Can you work these out from the model? Positions are in its coordinate system, mm. Coordinates: 2 decimals unless noted, no trailing zeros. Loops run counter-clockwise (first coordinate to the right, second up) from the corner with the lowest first, then second, coordinate; pieces in that order, holes last.
Autodesk Inventor part; units mm, degrees
ref_plane "BODYS_XY" through (0, 0, 0) normal (1, 0, 0) x (0, 0, -1)
ref_plane "BODYS_YZ" through (0, 0, 0) normal (0, 0, -1) x (0, 1, 0)
ref_plane "BODYS_ZX" through (0, 0, 0) normal (0, 1, 0) x (1, 0, 0)
sketch "__2" plane through (0, 0, 0) normal (1, 0, 0) x (0, 1, 0)
  arc A0 (0.5, 35.5) -> (0, 35) centre (0.5, 35) ccw
  line L0 (0, 35) -> (0, -35)
  arc A1 (0, -35) -> (0.5, -35.5) centre (0.5, -35) ccw
  line L1 (0.5, -35.5) -> (6.3099, -35.5)
  arc A2 (6.3099, -35.5) -> (8.274, -33.877) centre (6.3099, -33.5) ccw
  arc A3 (8.274, -33.877) -> (8.7, -31.581) centre (-167.9972, 0.0159) ccw
  line L2 (8.7, -31.581) -> (8.7, -29.75)
  line L3 (8.7, -29.75) -> (9.051, -29.547)
  arc A4 (9.051, -29.547) -> (9.051, 29.547) centre (-168.0005, 0) ccw
  line L4 (9.051, 29.547) -> (8.7, 29.75)
  line L5 (8.7, 29.75) -> (8.7, 31.581)
  arc A5 (8.7, 31.581) -> (8.274, 33.877) centre (-167.9972, -0.0159) ccw
  arc A6 (8.274, 33.877) -> (6.3099, 35.5) centre (6.3099, 33.5) ccw
  line L6 (6.3099, 35.5) -> (0.5, 35.5)
extrude "Extrusion1" add sketch "__2" along normal blind 597
sketch "__1" plane through (0, 7.18, 0) normal (0, 1, 0) x (1, 0, 0)
  circle A0 centre (8, 30.29) radius 3.25
extrude "Extrusion2" cut sketch "__1" along normal blind 3.52
pattern_linear "Rectangular Pattern1" count 2 spacing 631 along (1, 0, 0) count 2 spacing 60.58 along (0, 0, 1) of "Extrusion2"
ref_plane "BODYS_XY" through (0, 0, 0) normal (1, 0, 0) x (0, 0, -1)
ref_plane "BODYS_YZ" through (0, 0, 0) normal (0, 0, -1) x (0, 1, 0)
ref_plane "BODYS_ZX" through (0, 0, 0) normal (0, 1, 0) x (1, 0, 0)
properties part number "ETH2-17-350_3"
Item 1: Suppose I cut it at A-A, the plane x = 533. Please give me the cut outline in (y, z), plus the area to 3 significant figures.
Results are:
outline: (0, -35) arc R0.5 ccw to (0.5, -35.5) - (6.31, -35.5) arc R2 ccw to (8.27, -33.88) arc R179.5 ccw to (8.7, -31.58) - (8.7, -29.75) - (9.05, -29.55) arc R179.5 ccw to (9.05, 29.55) - (8.7, 29.75) - (8.7, 31.58) arc R179.5 ccw to (8.27, 33.88) arc R2 ccw to (6.31, 35.5) - (0.5, 35.5) arc R0.5 ccw to (0, 35) - close
area: 731 mm2
Item 2: I need wall thicknesses on line 1 along Y through (x, z) = (392.5, 11); line 2 along Z through (x, y) = (8, 7.9); line 3 along Y through (x, z) = (493.5, -3.5). Which ranges of each line are inside material? Lowest first, please.
Results are:
line 1: y = 0 to 11.16
line 2: z = -34.71 to -33.54, -27.04 to 27.04, 33.54 to 34.71
line 3: y = 0 to 11.47
Item 3: Suppose I cut it at B-B, the plane z = 9.5. Please give me the cut outline in (x, y).
Results are:
outline: (0, 0) - (597, 0) - (597, 11.25) - (0, 11.25) - close
Item 4: I'm going to push flat-ended pins straight in: P1, Ø2, axis at x = 404, z = 30.5, coming from the +Y side; P2, Ø0.5, axis at x = 1.5, z = -30.5, coming from the +Y side; P3, Ø10.5, axis at x = 8, z = -30.29, coming from the +Y side. Where does each tip first touch, or does it pass through?
Results are:
P1: stops at y = 9.06
P2: stops at y = 8.7
P3: stops at y = 9.74
